from build123d import *

# Parameters (mm, degrees)
EXTRUDE_1_DEPTH      = 850.470859
EXTRUDE_1_DEPTH_BACK = 15
SKETCH_3_R           = 12.6
CUT_EXTRUDE_1_DEPTH  = 31


with BuildPart() as part:
    # Эскиз2 → Бобышка-Вытянуть1 (new body, two sides)
    with BuildSketch(Plane(origin=(0, 0, 0), x_dir=(0, 0, -1), z_dir=(1, 0, 0))) as extrude_1_sk:
        with BuildLine():
            Line((-12, 30), (12, 30))
            ThreePointArc((12, 30), (14.121320344, 29.121320344), (15, 27))
            Line((15, 27), (15, 3))
            ThreePointArc((15, 3), (14.121320344, 0.878679656), (12, 0))
            Line((12, 0), (-12, 0))
            ThreePointArc((-12, 0), (-14.121320344, 0.878679656), (-15, 3))
            Line((-15, 3), (-15, 27))
            ThreePointArc((-15, 27), (-14.121320344, 29.121320344), (-12, 30))
        make_face()
        with BuildLine():
            Line((-11, 28), (11, 28))
            ThreePointArc((11, 28), (12.414213562, 27.414213562), (13, 26))
            Line((13, 26), (13, 4))
            ThreePointArc((13, 4), (12.414213562, 2.585786438), (11, 2))
            Line((11, 2), (-11, 2))
            ThreePointArc((-11, 2), (-12.414213562, 2.585786438), (-13, 4))
            Line((-13, 4), (-13, 26))
            ThreePointArc((-13, 26), (-12.414213562, 27.414213562), (-11, 28))
        make_face(mode=Mode.SUBTRACT)
    extrude(amount=EXTRUDE_1_DEPTH)
    extrude(extrude_1_sk.sketch, amount=-EXTRUDE_1_DEPTH_BACK)

    # Эскиз3 → Вырез-Вытянуть1 (cut, through all)
    with BuildSketch(Plane.XY.offset(15)):
        Circle(SKETCH_3_R)
        with Locations((278.490286217, 0)):
            Circle(SKETCH_3_R)
        with Locations((556.980572433, 0)):
            Circle(SKETCH_3_R)
        with Locations((835.47085865, 0)):
            Circle(SKETCH_3_R)
    extrude(amount=-CUT_EXTRUDE_1_DEPTH, mode=Mode.SUBTRACT)


solid = part.part
Can you work these out from the model? Positions are in its coordinate system, mm. A direction names the side the tool comes from. Coordinates: 2 decimals unless noted, no trailing zeros. Order: outer loops, then holes, each group sorted by start corner. A loop starts at its lowest first (then second) coordinate and runs counter-clockwise, first axis right, second up. Notation, with made-up numbers: (72, 65) - (91, 65) arc R16 ccw to (91, 75) - close; hole circle Ø4 at (9, -30.5). An arc over 180 degrees is marked (long way). Answer as a JSON object with one key per item and string values. Group by question number.
Q1. I need wall thicknesses on line 1 (Y direction, x = 350, z = 5); line 2 (Z direction, x = 793, y = 10); line 3 (Y direction, x = 25, z = 12.5). Which ranges of each line are inside material? Lowest first, please. Write a range as from..to.
Q2. Imagine slicing it at C-C (x = 0). Please give me the cut outline in (y, z).
Q3. On a 3-axis mill with a long thin cutter (end or side, diameter ignored), from which of +Z, -Z, +X, -X, +Y, -Y can I reach the whole of each face in a straight line? I mean faces 4 (the face through (698, 2, 0)), 5 (the face through (424, 15, 15)). Say none if no direction works.
Q4. We'd pull the mould along Z, two halves only. Please class faces 1 (the face through (420, 0, 0)), 2 (the face through (424, 15, -15)), 3 (the face through (424, 15, -13)): +Z half, -Z half, draft (parallel to the pull), parting line (faces both ways), or undercut.
Q5. Imagine slicing it at B-B (x = 310.5). Please give me the cut outline in (y, z), and give its area (3 significant figures).
Q6. Imagine slicing it at A-A (z = -3.5). Please give me the cut outline in (x, y).
Determined:
{
 "1": {"line 1": "y = 0..2, 28..30", "line 2": "z = -15..-13, 13..15", "line 3": "y = 0.04..2.68, 27.32..29.96"},
 "2": {"outline": "(12.6, -15) - (27, -15) arc R3 ccw to (30, -12) - (30, 12) arc R3 ccw to (27, 15) - (12.6, 15) - (12.6, 13) - (26, 13) arc R2 cw to (28, 11) - (28, -11) arc R2 cw to (26, -13) - (12.6, -13) - close"},
 "3": {"face 4": "+X, -X", "face 5": "+Z, +X, -X, +Y, -Y"},
 "4": {"face 1": "draft", "face 2": "-Z half", "face 3": "undercut"},
 "5": {"outline": "(0, -12) arc R3 ccw to (3, -15) - (27, -15) arc R3 ccw to (30, -12) - (30, 12) arc R3 ccw to (27, 15) - (3, 15) arc R3 ccw to (0, 12) - close; hole (2, -11) arc R2 ccw to (4, -13) - (26, -13) arc R2 ccw to (28, -11) - (28, 11) arc R2 ccw to (26, 13) - (4, 13) arc R2 ccw to (2, 11) - close", "area": "220 mm2"},
 "6": {"outline": "(-15, 0) - (-12.6, 0) arc R12.6 cw to (-12.44, 2) - (-15, 2) - close; (-15, 28) - (850.47, 28) - (850.47, 30) - (-15, 30) - close; (12.44, 2) arc R12.6 cw to (12.6, 0) - (265.89, 0) arc R12.6 cw to (266.05, 2) - close; (290.93, 2) arc R12.6 cw to (291.09, 0) - (544.38, 0) arc R12.6 cw to (544.54, 2) - close; (569.42, 2) arc R12.6 cw to (569.58, 0) - (822.87, 0) arc R12.6 cw to (823.03, 2) - close; (847.91, 2) arc R12.6 cw to (848.07, 0) - (850.47, 0) - (850.47, 2) - close"}
}
